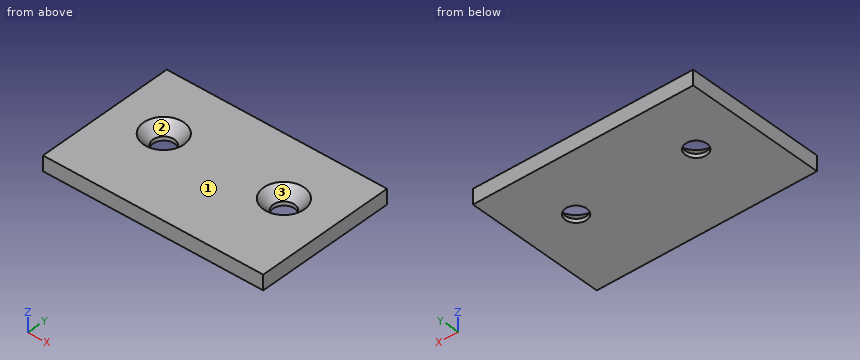
```python
from build123d import *

# Parameters (mm, degrees)
SKETCH1_W                                     = 69.85
SKETCH1_H                                     = 44.45
BOSS_EXTRUDE1_DEPTH                           = 4.7498
CSK_FOR_1_4_FLAT_HEAD_MACHINE_SCREW1_AT_COUNT = 2
CSK_FOR_1_4_FLAT_HEAD_MACHINE_SCREW1_AT_PITCH = 38.1


with BuildPart() as part:
    # Sketch1 → Boss-Extrude1 (new body)
    with BuildSketch(Plane.XY):
        with Locations((0, 22.225)):
            Rectangle(SKETCH1_W, SKETCH1_H)
    extrude(amount=BOSS_EXTRUDE1_DEPTH)

    # Sketch3 → CSK for 1/4 Flat Head Machine Screw1 (revolve, cut)
    with BuildSketch(Plane(origin=(19.05, 25.4, 4.7498), x_dir=(0, -1, 0), z_dir=(1, 0, 0))):
        Polygon((0, 0), (0, 4.7498), (3.3782, 4.7498), (3.3782, 3.520932584), (6.4389, 0), align=None)
    csk_for_1_4_flat_head_machine_screw1 = revolve(axis=Axis((19.05, 25.4, 11.0998), (0, 0, -1)), mode=Mode.SUBTRACT)

    # CSK for 1/4 Flat Head Machine Screw1 at: CSK for 1/4 Flat Head Machine Screw1 ×2
    with Locations(*[(-i * CSK_FOR_1_4_FLAT_HEAD_MACHINE_SCREW1_AT_PITCH, 0, 0) for i in range(1, CSK_FOR_1_4_FLAT_HEAD_MACHINE_SCREW1_AT_COUNT)]):
        add(csk_for_1_4_flat_head_machine_screw1, mode=Mode.SUBTRACT)


solid = part.part
```
Design review of the part built by this model. Coordinates are the model's own, in mm. Face numbers are marked on the shaded views. Give positions to 0.01 mm unless a question says otherwise; leave off trailing zeros. Order: outer loops, then holes, each group sorted by start corner. A loop starts at its lowest first (then second) coordinate and runs counter-clockwise, first axis right, second up. Notation, with made-up numbers: (72.5, 87) - (83.5, 87) arc R35 cw to (83.5, 121) - close; hole circle Ø11 at (10.5, 75). An arc over 180 degrees is marked (long way). Use a Markdown table: item, result. Add a question column.
(1) Add section B-B on x = 19.05. Give the boundary of the cut face in (y, z).
(2) Add section C-C on z = 3. Give the boundary of the cut face in (x, y) (3 decimals).
(3) Clearance check with a flat-ended pin moving along its axis: P1, Ø11, axis at x = 19.05, y = 25.4, coming from the +Z side. State where the tip first meets the part, or that it passes through.
(4) Add section A-A on y = 25.4. Give the boundary of the cut face in (x, z) (3 decimals).
(5) Wall thickness on probe 1 along X at (y, z) = (25.4, 0.55) (3 decimals); probe 2 along Y at (x, z) = (-19.05, 0.55); probe 3 along X at (y, z) = (26, 4.2) (3 decimals): over which ranges is each line inside the solid? List them lowest first. Write a range as [from, to].
(6) Mouldability with a two-part tool opening along Y and no side actions: class the marked faces 1, 2 and 3 as +Y half, -Y half, draft (parallel to the pull), parting line (faces both ways), or undercut.
Report:
| question | item | result |
|---|---|---|
| 1 | outline | (0, 0) - (22.02, 0) - (22.02, 1.23) - (18.96, 4.75) - (0, 4.75) - close; (28.78, 0) - (44.45, 0) - (44.45, 4.75) - (31.84, 4.75) - (28.78, 1.23) - close |
| 2 | outline | (-34.925, 0) - (34.925, 0) - (34.925, 44.45) - (-34.925, 44.45) - close; hole circle Ø9.836 at (-19.05, 25.4); hole circle Ø9.836 at (19.05, 25.4) |
| 3 | P1 | stops at z = 3.67 |
| 4 | outline | (-34.925, 0) - (-22.428, 0) - (-22.428, 1.229) - (-25.489, 4.75) - (-34.925, 4.75) - close; (-15.672, 0) - (15.672, 0) - (15.672, 1.229) - (12.611, 4.75) - (-12.611, 4.75) - (-15.672, 1.229) - close; (22.428, 0) - (34.925, 0) - (34.925, 4.75) - (25.489, 4.75) - (22.428, 1.229) - close |
| 5 | probe 1 | x = [-34.925, -22.428], [-15.672, 15.672], [22.428, 34.925] |
| 5 | probe 2 | y = [0, 22.02], [28.78, 44.45] |
| 5 | probe 3 | x = [-34.925, -24.981], [-13.119, 13.119], [24.981, 34.925] |
| 6 | face 1 | draft |
| 6 | face 2 | undercut |
| 6 | face 3 | undercut |
